```python
from build123d import *

# Parameters (mm, degrees)
F1_DEPTH = 12
F2_R     = 5
F2_R_2   = 4.5
F3_DEPTH = 10
F4_R     = 6
F4_R_2   = 4.5
F5_DEPTH = 1
F6_DEPTH = 25
F7_SIZE  = 0.5


with BuildPart() as f1:
    # F0 (on Front) → F1 (new body)
    with BuildSketch(Plane.XZ):
        with BuildLine():
            Line((-5.8526312746, -17.3661426386), (-5.8526312746, 22.4338573614))
            ThreePointArc((-5.8526312746, 22.4338573614), (-5.8672759356, 22.4692127005), (-5.9026312746, 22.4838573614))
            Line((-5.9026312746, 22.4838573614), (-7.1112099184, 22.4838573614))
            ThreePointArc((-7.1112099184, 22.4838573614), (-7.157403895, 22.452991533), (-7.1465652574, 22.3985020224))
            Line((-7.1465652574, 22.3985020224), (-6.8172759356, 22.0692127005))
            ThreePointArc((-6.8172759356, 22.0692127005), (-6.806437298, 22.0147231898), (-6.8526312746, 21.9838573614))
            Line((-6.8526312746, 21.9838573614), (-7.8526312746, 21.9838573614))
            Line((-7.8526312746, 21.9838573614), (-7.8526312746, -16.9161426386))
            Line((-7.8526312746, -16.9161426386), (-6.8526312746, -16.9161426386))
            ThreePointArc((-6.8526312746, -16.9161426386), (-6.806437298, -16.947008467), (-6.8172759356, -17.0014979776))
            Line((-6.8172759356, -17.0014979776), (-7.1465652574, -17.3307872995))
            ThreePointArc((-7.1465652574, -17.3307872995), (-7.157403895, -17.3852768102), (-7.1112099184, -17.4161426386))
            Line((-7.1112099184, -17.4161426386), (-5.9026312746, -17.4161426386))
            ThreePointArc((-5.9026312746, -17.4161426386), (-5.8672759356, -17.4014979776), (-5.8526312746, -17.3661426386))
        make_face()
    extrude(amount=F1_DEPTH)

    # F2 (on face) → F3 (join)
    with BuildSketch(Plane(origin=(-7.8526312746, 0, 0), x_dir=(0, -1, 0), z_dir=(-1, 0, 0))):
        with Locations((6, 12.5338573614)):
            Circle(F2_R)
        with Locations((6, 12.5338573614)):
            Circle(F2_R_2, mode=Mode.SUBTRACT)
        with Locations((6, -7.4661426386)):
            Circle(F2_R)
        with Locations((6, -7.4661426386)):
            Circle(F2_R_2, mode=Mode.SUBTRACT)
    extrude(amount=F3_DEPTH)

    # F4 (on face) → F5 (join)
    with BuildSketch(Plane(origin=(-17.8526312746, 0, 0), x_dir=(0, -1, 0), z_dir=(-1, 0, 0))):
        with Locations((6, 12.5338573614)):
            Circle(F4_R)
        with Locations((6, 12.5338573614)):
            Circle(F4_R_2, mode=Mode.SUBTRACT)
        with Locations((6, -7.4661426386)):
            Circle(F4_R)
        with Locations((6, -7.4661426386)):
            Circle(F4_R_2, mode=Mode.SUBTRACT)
    extrude(amount=F5_DEPTH)

    # F6 (cut): faces of the model
    f6_faces = [f1.faces().sort_by_distance(p)[0] for p in [
        (-7.8526312746, -6, 12.5338573614),
        (-7.8526312746, -6, -7.4661426386),
    ]]
    extrude(f6_faces, amount=-F6_DEPTH, mode=Mode.SUBTRACT)

    # F7
    f7_edges = [f1.edges().sort_by_distance(p)[0] for p in [
        (-18.852631, 0, 12.533857),
        (-18.852631, 0, -7.466143),
    ]]
    chamfer(f7_edges, length=F7_SIZE)


solid = f1.part
```
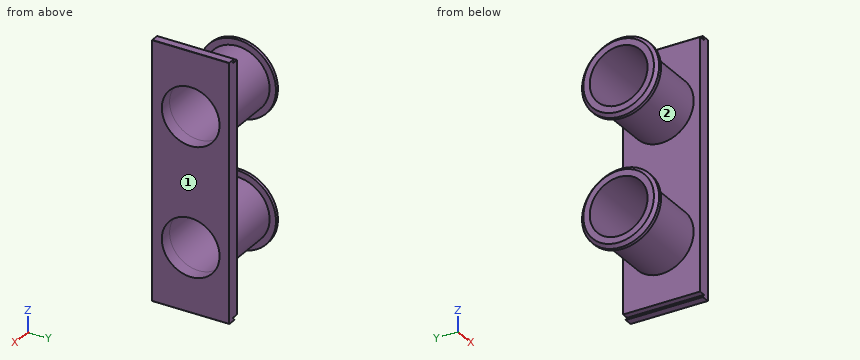
CAD build for the part. Positions are in the model's coordinates, mm. Face numbers are marked on the shaded views. Coordinates: 2 decimals unless noted, no trailing zeros. Order: outer loops, then holes, each group sorted by start corner. A loop starts at its lowest first (then second) coordinate and runs counter-clockwise, first axis right, second up. Notation, with made-up numbers: (-26, 76.25) - (26, 76.25) arc R24 cw to (26, 88.25) - close; hole circle Ø7 at (-34, 3.5). An arc over 180 degrees is marked (long way). Use a Markdown table: item, result. Add a question column.
(1) Saw through at B-B (y = -6). Count the separate pieces of the cut face and the enclosed holes in it, then the cut area to 3 significant figures.
(2) Saw through at A-A (x = -8.25). Give the cut face in (y, z), then the cut area to 3 significant figures.
(3) Pull direction X, two halves, no side cores. Call the marked faces 1 and 2: +X half, -X half, draft (parallel to the pull), parting line (faces both ways), or undercut.
(4) Saw through at C-C (z = 1.5). Give the cut face in (x, y), then the cut area to 3 significant figures.
(5) Flat gauge pins, fed straight in: pin 1 (2 mm diameter, centred on x = -12, y = -8, fed in from -Z); pin 2 (0.5 mm diameter, centred on x = -7.5, y = -9, fed in from -Z); pin 3 (4 mm diameter, centred on x = -10, z = -6.5, fed in from -Y); pin 4 (5 mm diameter, centred on y = -4.5, z = 12, fed in from -X). Where does each tip first touch, or does it go through?
(6) Drill centre lines: line 1 along Z through (x, y) = (-7.5, -6); line 2 along Z through (x, y) = (-13.5, -6); line 3 along Z through (x, y) = (-13.75, -7.75). Where is each one in solid material? Low to high. Write a range as [from, to].
Solved:
| question | item | result |
|---|---|---|
| 1 | separate pieces | 3 |
| 1 | enclosed holes | 0 |
| 1 | area | 68.4 mm² |
| 2 | outline | circle Ø10 at (-6, -7.47); circle Ø10 at (-6, 12.53); hole circle Ø9 at (-6, -7.47); hole circle Ø9 at (-6, 12.53) |
| 2 | area | 29.8 mm² |
| 3 | face 1 | +X half |
| 3 | face 2 | undercut |
| 4 | outline | (-7.85, -12) - (-5.85, -12) - (-5.85, 0) - (-7.85, 0) - close |
| 4 | area | 24.0 mm² |
| 5 | pin 1 | stops at z = -12.37 |
| 5 | pin 2 | stops at z = -16.92 |
| 5 | pin 3 | stops at y = -11 |
| 5 | pin 4 | passes through |
| 6 | line 1 | z = [-16.92, -11.97], [-2.97, 8.03], [17.03, 21.98] |
| 6 | line 2 | z = [-12.47, -11.97], [-2.97, -2.47], [7.53, 8.03], [17.03, 17.53] |
| 6 | line 3 | z = [-12.15, -11.61], [-3.32, -2.78], [7.85, 8.39], [16.68, 17.22] |
